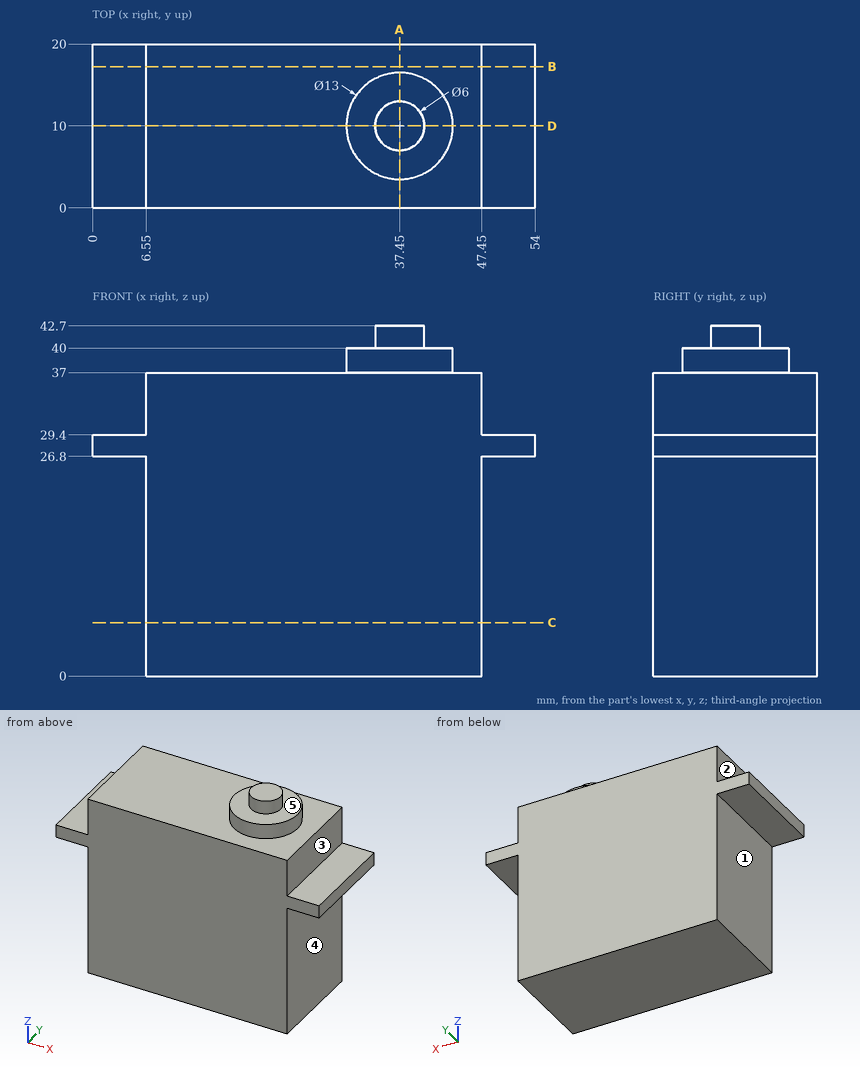
Geometry check sheet. Reference: drawing and pictorial views, mm from the part's lowest x, y, z. A direction names the side the tool comes from. Round coordinates to 2 decimals unless told otherwise and drop trailing zeros. Write each loop counter-clockwise with the first axis right and the second up, starting at its lowest first coordinate (ties: lowest second). Pieces come first, ordered by that corner, then holes.
Item 1: Section check D-D (y = 10). Record the boundary of the cut face in (x, z), plus the area to 3 significant figures.
Determined:
outline: (0, 26.8) - (6.55, 26.8) - (6.55, 0) - (47.45, 0) - (47.45, 26.8) - (54, 26.8) - (54, 29.4) - (47.45, 29.4) - (47.45, 37) - (43.95, 37) - (43.95, 40) - (40.45, 40) - (40.45, 42.7) - (34.45, 42.7) - (34.45, 40) - (30.95, 40) - (30.95, 37) - (6.55, 37) - (6.55, 29.4) - (0, 29.4) - close
area: 1,600 mm2
Item 2: Go/stop test with flat-tipped pins: pin 1 Ø7 at (x, y) = (2.5, 7) entering from +Z; pin 2 Ø2 at (x, y) = (49, 11) entering from -Z; pin 3 Ø10 at (y, z) = (5.5, 7.5) entering from -X. Record where each tip stops, or that it passes through.
Determined:
pin 1: stops at z = 29.4
pin 2: stops at z = 26.8
pin 3: stops at x = 6.55
Item 3: Section check B-B (y = 17.25). Record the boundary of the cut face in (x, z).
Determined:
outline: (0, 26.8) - (6.55, 26.8) - (6.55, 0) - (47.45, 0) - (47.45, 26.8) - (54, 26.8) - (54, 29.4) - (47.45, 29.4) - (47.45, 37) - (6.55, 37) - (6.55, 29.4) - (0, 29.4) - close
Item 4: Section check A-A (x = 37.45). Record the boundary of the cut face in (y, z), plus the area to 3 significant figures.
Determined:
outline: (0, 0) - (20, 0) - (20, 37) - (16.5, 37) - (16.5, 40) - (13, 40) - (13, 42.7) - (7, 42.7) - (7, 40) - (3.5, 40) - (3.5, 37) - (0, 37) - close
area: 795 mm2
Item 5: Section check C-C (z = 6.5). Record the boundary of the cut face in (x, y).
Determined:
outline: (6.55, 0) - (47.45, 0) - (47.45, 20) - (6.55, 20) - close
Item 6: Material ranges on line 1 along X through (y, z) = (12, 13); line 2 along Z through (x, y) = (30, 17.25); line 3 along Z through (x, y) = (51, 12), recorded low to high.
Determined:
line 1: x = 6.55 to 47.45
line 2: z = 0 to 37
line 3: z = 26.8 to 29.4
Item 7: Access from +Z, -Z, +X, -X, +Y, -Y to the whole of each face (thin tool, end or side, straight path). Record for the marked faces 1, 2, 3, 4 and 5.
Determined:
face 1: -Z, -X, +Y, -Y
face 2: +Z, -X, +Y, -Y
face 3: +Z, +X, +Y, -Y
face 4: -Z, +X, +Y, -Y
face 5: +Z
